Autodesk Inventor part; units mm, degrees
ref_plane "YZ Plane" through (0, 0, 0) normal (1, 0, 0) x (0, 1, 0)
ref_plane "XZ Plane" through (0, 0, 0) normal (0, 1, 0) x (-1, 0, 0)
ref_plane "XY Plane" through (0, 0, 0) normal (0, 0, 1) x (1, 0, 0)
sketch "Sketch1" plane through (0, 0, 0) normal (0, 0, 1) x (1, 0, 0)
  line L0 (-18.0179, 30.122) -> (11.7821, 30.122)
  line L1 (11.7821, 30.122) -> (11.7821, -21.278)
  line L2 (11.7821, -21.278) -> (-18.0179, -21.278)
  line L3 (-18.0179, -21.278) -> (-18.0179, 30.122)
  point P0 (0, 0)
  dimension "d0" = 29.8
  dimension "d1" = 51.4
extrude "Extrusion1" add sketch "Sketch1" along normal blind 2
sketch "Sketch2" plane through (0, 0, 2) normal (0, 0, 1) x (1, 0, 0)
  line L0 (-18.0179, 30.122) -> (11.7821, 30.122)
  line L1 (11.7821, 30.122) -> (11.7821, -21.278)
  line L2 (11.7821, -21.278) -> (-18.0179, -21.278)
  line L3 (-18.0179, -21.278) -> (-18.0179, 30.122)
  line L4 (-16.0179, 28.122) -> (9.7821, 28.122)
  line L5 (9.7821, 28.122) -> (9.7821, -19.278)
  line L6 (9.7821, -19.278) -> (-16.0179, -19.278)
  line L7 (-16.0179, -19.278) -> (-16.0179, 28.122)
  point P0 (0, 0)
  dimension "d4" = 2
  dimension "d5" = 2
  dimension "d6" = 2
  dimension "d7" = 2
  dimension "d8" = 25.8
  dimension "d9" = 47.4
extrude "Extrusion2" add sketch "Sketch2" along normal blind 6
sketch "Sketch3" plane through (0, 0, 2) normal (0, 0, 1) x (1, 0, 0)
  point P0 (0, 0)
sketch "Sketch4" plane through (0, 0, 2) normal (0, 0, 1) x (1, 0, 0)
  line L0 (-18.0179, 30.122) -> (-10.0179, 30.122)
  line L1 (-10.0179, 30.122) -> (-10.0179, 22.122)
  line L2 (-10.0179, 22.122) -> (-18.0179, 22.122)
  line L3 (-18.0179, 22.122) -> (-18.0179, 30.122)
  line L4 (11.7821, 30.122) -> (3.7821, 30.122)
  line L5 (3.7821, 30.122) -> (3.7821, 22.122)
  line L6 (3.7821, 22.122) -> (11.7821, 22.122)
  line L7 (11.7821, 22.122) -> (11.7821, 30.122)
  line L8 (-18.0179, -21.278) -> (-10.0179, -21.278)
  line L9 (-10.0179, -21.278) -> (-10.0179, -13.278)
  line L10 (-10.0179, -13.278) -> (-18.0179, -13.278)
  line L11 (-18.0179, -13.278) -> (-18.0179, -21.278)
  line L12 (11.7821, -21.278) -> (3.7821, -21.278)
  line L13 (3.7821, -21.278) -> (3.7821, -13.278)
  line L14 (3.7821, -13.278) -> (11.7821, -13.278)
  line L15 (11.7821, -13.278) -> (11.7821, -21.278)
  line L16 (-18.0179, 30.122) -> (-18.0179, -21.278)
  line L17 (-18.0179, -21.278) -> (11.7821, -21.278)
  point P0 (0, 0)
  dimension "d12" = 8
  dimension "d13" = 8
  dimension "d14" = 8
  dimension "d15" = 8
  dimension "d16" = 8
  dimension "d17" = 8
  dimension "d18" = 8
  dimension "d19" = 8
  dimension "d20" = 35.4
extrude "Extrusion3" add sketch "Sketch4" along normal blind 6
sketch "Sketch5" plane through (0, 0, 2) normal (0, 0, 1) x (1, 0, 0)
  line L0 (9.7821, 22.122) -> (9.7821, -13.278)
  line L1 (-16.0179, 22.122) -> (9.7821, 22.122)
  line L2 (9.7821, 22.122) -> (9.7821, 20.122)
  line L3 (9.7821, 20.122) -> (-16.0179, 20.122)
  line L4 (-16.0179, 20.122) -> (-16.0179, 22.122)
  line L5 (-16.0179, -13.278) -> (9.7821, -13.278)
  line L6 (9.7821, -13.278) -> (9.7821, -11.278)
  line L7 (9.7821, -11.278) -> (-16.0179, -11.278)
  line L8 (-16.0179, -11.278) -> (-16.0179, -13.278)
  point P0 (0, 0)
  dimension "d23" = 2
  dimension "d24" = 2
extrude "Extrusion4" add sketch "Sketch5" along normal blind 2
sketch "Sketch6" plane through (0, 0, 8) normal (0, 0, 1) x (1, 0, 0)
  point P0 (0, 0)
sketch "Sketch7" plane through (0, 0, 8) normal (0, 0, 1) x (1, 0, 0)
  line L0 (-10.0179, -13.278) -> (-16.0179, -13.278)
  line L1 (-18.0179, 30.122) -> (-18.0179, -21.278)
  line L2 (9.7821, -13.278) -> (3.7821, -13.278)
  line L3 (11.7821, 30.122) -> (11.7821, -21.278)
  line L4 (11.7821, 30.122) -> (-18.0179, 30.122)
  point P0 (0, 0)
  point P1 (-14.0179, 26.122)
  point P2 (7.7821, 26.122)
  point P3 (-14.0179, -17.278)
  point P4 (7.7821, -17.278)
  dimension "d27" = 4
  dimension "d28" = 4
  dimension "d29" = 4
  dimension "d30" = 4
  dimension "d31" = 4
  dimension "d32" = 4
  dimension "d33" = 4
  dimension "d34" = 4
hole "Hole1" at (-14.0179, 26.122, 8) at (7.7821, 26.122, 8) at (-14.0179, -17.278, 8) at (7.7821, -17.278, 8) direction (0, 0, -1) diameter 3 depth 6 tip angle 118
fillet "Fillet1" radius 3 4 edges at (-18.0179, -21.278, 4) (11.7821, -21.278, 4) (-18.0179, 30.122, 4) (11.7821, 30.122, 4)
sketch "Sketch8" plane through (0, 0, 8) normal (0, 0, 1) x (1, 0, 0)
  line L0 (9.7821, 22.122) -> (9.7821, -13.278)
  line L1 (-16.0179, -13.278) -> (-16.0179, 22.122)
  point P0 (0, 0)
  dimension "d43" = 25.8
properties part number "base"
Verification items for the finished model (mm, model axes). A direction names the side the tool comes from. Round coordinates to 2 decimals unless told otherwise and drop trailing zeros. Loops run counter-clockwise (first coordinate to the right, second up) from the corner with the lowest first, then second, coordinate; pieces in that order, holes last. Notation, with made-up numbers: (84, -2.5) - (96, -2.5) arc R13 ccw to (96, 18.5) - close; hole circle Ø8 at (14.25, 6). An arc over 180 degrees is marked (long way). Use one line per item in the form item = value.
1. Section check D-D on x = -0.25. Record the cut outline in (y, z), and give its area (3 significant figures).
A:
outline = (-21.28, 0) - (30.12, 0) - (30.12, 8) - (28.12, 8) - (28.12, 2) - (22.12, 2) - (22.12, 4) - (20.12, 4) - (20.12, 2) - (-11.28, 2) - (-11.28, 4) - (-13.28, 4) - (-13.28, 2) - (-19.28, 2) - (-19.28, 8) - (-21.28, 8) - close
area = 135 mm²
2. Draft check along X on faces 1 (the cylindrical face through (-17.116, 29.267, 4.056)), 2 (the flat face through (7, 22.122, 6)), 3 (the flat face through (-3, -21.278, 4)), 4 (the flat face through (-3, 21, 4)). Enter one of: pulls with the +X half, pulls with the -X half, needs draft (parallel to the pull), parting line crosses it, or undercut.
A:
face_1 = pulls with the -X half
face_2 = undercut
face_3 = needs draft
face_4 = undercut
3. Gauge pin test, flat ends, axial feed: pin 1 Ø5 at (x, y) = (1, 7) entering from -Z; pin 2 Ø1.5 at (x, y) = (2.5, 19.5) entering from +Z; pin 3 Ø10 at (x, y) = (-4.5, -2) entering from +Z. Record the tip position at first contact, or that the pin passes through.
A:
pin_1 = 0
pin_2 = 4
pin_3 = 2
4. Scan lines: probe 1 along X at (y, z) = (20.5, 6.75); probe 2 along Y at (x, z) = (-14, 4.25); probe 3 along Y at (x, z) = (-3.5, 6.5). Record each from-to range of solid material in increasing order.
A:
probe_1 = -18.02 to -16.02, 9.78 to 11.78
probe_2 = -21.28 to -18.78, -15.78 to -13.28, 22.12 to 24.62, 27.62 to 30.12
probe_3 = -21.28 to -19.28, 28.12 to 30.12
5. Access from +Z, -Z, +X, -X, +Y, -Y to the whole of each face (thin tool, end or side, straight path). Record for faces 5 (the cylindrical face through (-17.16, -20.38, 4.06)), 6 (the flat face through (-10.018, 25, 5)).
A:
face_5 = +Z, -Z, -X, -Y
face_6 = +Z
6. Section check C-C on y = -9.5. Record the cut outline in (x, z), and give its area (3 significant figures).
A:
outline = (-18.02, 0) - (11.78, 0) - (11.78, 8) - (9.78, 8) - (9.78, 2) - (-16.02, 2) - (-16.02, 8) - (-18.02, 8) - close
area = 83.6 mm²
7. Section check B-B on x = -12. Record the cut outline in (y, z).
A:
outline = (-21.28, 0) - (30.12, 0) - (30.12, 8) - (22.12, 8) - (22.12, 4) - (20.12, 4) - (20.12, 2) - (-11.28, 2) - (-11.28, 4) - (-13.28, 4) - (-13.28, 8) - (-21.28, 8) - close
8. Section check A-A on z = 5.5. Record the cut outline in (x, y).
A:
outline = (-18.02, -18.28) arc R3 ccw to (-15.02, -21.28) - (8.78, -21.28) arc R3 ccw to (11.78, -18.28) - (11.78, 27.12) arc R3 ccw to (8.78, 30.12) - (-15.02, 30.12) arc R3 ccw to (-18.02, 27.12) - close; hole (-16.02, -13.28) - (-10.02, -13.28) - (-10.02, -19.28) - (3.78, -19.28) - (3.78, -13.28) - (9.78, -13.28) - (9.78, 22.12) - (3.78, 22.12) - (3.78, 28.12) - (-10.02, 28.12) - (-10.02, 22.12) - (-16.02, 22.12) - close; hole circle Ø3 at (-14.02, -17.28); hole circle Ø3 at (-14.02, 26.12); hole circle Ø3 at (7.78, -17.28); hole circle Ø3 at (7.78, 26.12)
